The listing builds one solid part. Answer for the finished solid, in the listing's coordinates (mm). A direction names the side the tool comes from. Coordinates: 2 decimals unless noted, no trailing zeros. Write each loop counter-clockwise with the first axis right and the second up, starting at its lowest first coordinate (ties: lowest second). Pieces come first, ordered by that corner, then holes.
from build123d import *

# Parameters (mm, degrees)
SKETCH1_W               = 70.4
SKETCH1_H               = 2
BOSS_EXTRUDE2_DEPTH     = 10
SKETCH2_W               = 2
SKETCH2_H               = 55
BOSS_EXTRUDE3_DEPTH     = 10
SKETCH3_W               = 19
SKETCH3_H               = 3
BOSS_EXTRUDE4_DEPTH     = 2
SKETCH4_W               = 15
SKETCH4_H               = 10
CUT_EXTRUDE2_DEPTH      = 2
SKETCH5_W               = 2
SKETCH5_H               = 3
BOSS_EXTRUDE5_DEPTH     = 1
SKETCH6_W               = 2
SKETCH6_H               = 3
BOSS_EXTRUDE6_DEPTH     = 1
SKETCH7_W               = 57
SKETCH7_H               = 2
BOSS_EXTRUDE7_DEPTH     = 6.6
SKETCH8_W               = 57
SKETCH8_H               = 2
BOSS_EXTRUDE8_DEPTH     = 6.6
BOSS_EXTRUDE9_DEPTH     = 5
SKETCH12_W              = 2
SKETCH12_H              = 5
SKETCH12_H_2            = 40
SKETCH12_H_3            = 30
BOSS_EXTRUDE10_DEPTH    = 20
BOSS_EXTRUDE11_DEPTH    = 3
SKETCH14_W              = 0.5
SKETCH14_H              = 9
CUT_EXTRUDE3_DEPTH      = 3
SKETCH15_W              = 38.4
SKETCH15_H              = 45
CUT_EXTRUDE4_DEPTH      = 3
BOSS_EXTRUDE12_DEPTH    = 0.5
SKETCH17_R              = 1.8
SKETCH17_W              = 3
SKETCH17_H              = 5
CUT_EXTRUDE6_DEPTH      = 3
CUT_EXTRUDE8_DEPTH      = 32
CUT_EXTRUDE8_DEPTH_BACK = 49
SKETCH19_W              = 94.558020587
SKETCH19_H              = 51.225034616
CUT_EXTRUDE9_DEPTH      = 93
CUT_EXTRUDE9_DEPTH_BACK = 18
SKETCH20_W              = 91.945359737
SKETCH20_H              = 40.424662202
SKETCH21_W              = 45
SKETCH21_H              = 3
BOSS_EXTRUDE14_DEPTH    = 2.5
SKETCH22_W              = 2.5
SKETCH22_H              = 45
BOSS_EXTRUDE15_DEPTH    = 8
SKETCH23_R              = 1.8
CUT_EXTRUDE10_DEPTH     = 10


with BuildPart() as part:
    # Sketch1 → Boss-Extrude2 (new body)
    with BuildSketch(Plane(origin=(0, 0, 0), x_dir=(1, 0, 0), z_dir=(0, 1, 0))):
        with Locations((35.2, 1)):
            Rectangle(SKETCH1_W, SKETCH1_H)
    extrude(amount=BOSS_EXTRUDE2_DEPTH)

    # Sketch2 → Boss-Extrude3 (add)
    with BuildSketch(Plane(origin=(0, 10, 0), x_dir=(1, 0, 0), z_dir=(0, 1, 0))):
        with Locations((1, 29.5)):
            Rectangle(SKETCH2_W, SKETCH2_H)
        with Locations((69.4, 29.5)):
            Rectangle(SKETCH2_W, SKETCH2_H)
    extrude(amount=-BOSS_EXTRUDE3_DEPTH)

    # Sketch3 → Boss-Extrude4 (add)
    with BuildSketch(Plane.XY):
        with Locations((35.2, 11.5)):
            Rectangle(SKETCH3_W, SKETCH3_H)
    extrude(amount=-BOSS_EXTRUDE4_DEPTH)

    # Sketch4 → Cut-Extrude2 (cut)
    with BuildSketch(Plane.XY):
        with Locations((35.2, 5)):
            Rectangle(SKETCH4_W, SKETCH4_H)
    extrude(amount=-CUT_EXTRUDE2_DEPTH, mode=Mode.SUBTRACT)

    # Sketch5 → Boss-Extrude5 (add)
    with BuildSketch(Plane.ZY.offset(-25.7)):
        with Locations((-1, 11.5)):
            Rectangle(SKETCH5_W, SKETCH5_H)
    extrude(amount=BOSS_EXTRUDE5_DEPTH)

    # Sketch6 → Boss-Extrude6 (add)
    with BuildSketch(Plane(origin=(44.7, 0, 0), x_dir=(0, 0, -1), z_dir=(1, 0, 0))):
        with Locations((1, 11.5)):
            Rectangle(SKETCH6_W, SKETCH6_H)
    extrude(amount=BOSS_EXTRUDE6_DEPTH)

    # Sketch7 → Boss-Extrude7 (add)
    with BuildSketch(Plane.ZY):
        with Locations((-28.5, 1)):
            Rectangle(SKETCH7_W, SKETCH7_H)
    extrude(amount=BOSS_EXTRUDE7_DEPTH)

    # Sketch8 → Boss-Extrude8 (add)
    with BuildSketch(Plane(origin=(70.4, 0, 0), x_dir=(0, 0, -1), z_dir=(1, 0, 0))):
        with Locations((28.5, 1)):
            Rectangle(SKETCH8_W, SKETCH8_H)
    extrude(amount=BOSS_EXTRUDE8_DEPTH)

    # Sketch10 → Boss-Extrude9 (add)
    with BuildSketch(Plane(origin=(0, 0, -57), x_dir=(-1, 0, 0), z_dir=(0, 0, -1))):
        Polygon((-2, 10), (-2, 0), (6.6, 0), (6.6, 2), (0, 2), (0, 10), align=None)
        Polygon((-77, 0), (-68.4, 0), (-68.4, 10), (-70.4, 10), (-70.4, 2), (-77, 2), align=None)
    extrude(amount=BOSS_EXTRUDE9_DEPTH)

    # Sketch12 → Boss-Extrude10 (add)
    with BuildSketch(Plane(origin=(0, 10, 0), x_dir=(1, 0, 0), z_dir=(0, 1, 0))):
        with Locations((1, 59.5)):
            Rectangle(SKETCH12_W, SKETCH12_H)
        with Locations((1, 37)):
            Rectangle(SKETCH12_W, SKETCH12_H_2)
        with Locations((69.4, 42)):
            Rectangle(SKETCH12_W, SKETCH12_H_3)
        with Locations((69.4, 59.5)):
            Rectangle(SKETCH12_W, SKETCH12_H)
    extrude(amount=BOSS_EXTRUDE10_DEPTH)

    # Sketch13 → Boss-Extrude11 (add)
    with BuildSketch(Plane(origin=(0, 30, 0), x_dir=(1, 0, 0), z_dir=(0, 1, 0))):
        Polygon((0, 17), (35.2, 17), (35.2, 27), (70.4, 27), (70.4, 62), (0, 62), align=None)
    extrude(amount=BOSS_EXTRUDE11_DEPTH)

    # Sketch14 → Cut-Extrude3 (cut)
    with BuildSketch(Plane(origin=(0, 33, 0), x_dir=(1, 0, 0), z_dir=(0, 1, 0))):
        with Locations((11.7, 51)):
            Rectangle(SKETCH14_W, SKETCH14_H)
        with Locations((11.7, 38)):
            Rectangle(SKETCH14_W, SKETCH14_H)
        with Locations((11.7, 25.5)):
            Rectangle(SKETCH14_W, SKETCH14_H)
        with Locations((58.2, 51)):
            Rectangle(SKETCH14_W, SKETCH14_H)
        with Locations((58.2, 38)):
            Rectangle(SKETCH14_W, SKETCH14_H)
    extrude(amount=-CUT_EXTRUDE3_DEPTH, mode=Mode.SUBTRACT)

    # Sketch15 → Cut-Extrude4 (cut)
    with BuildSketch(Plane(origin=(0, 33, 0), x_dir=(1, 0, 0), z_dir=(0, 1, 0))):
        with Locations((35.2, 39.5)):
            Rectangle(SKETCH15_W, SKETCH15_H)
    extrude(amount=-CUT_EXTRUDE4_DEPTH, mode=Mode.SUBTRACT)

    # Sketch16 → Boss-Extrude12 (add)
    with BuildSketch(Plane.XY):
        Polygon((-6.6, 0), (27.7, 0), (27.7, 10), (42.7, 10), (42.7, 0), (77, 0), (77, 2), (70.4, 2), (70.4, 10), (45.7, 10), (45.7, 13), (24.7, 13), (24.7, 10), (0, 10), (0, 2), (-6.6, 2), align=None)
    extrude(amount=BOSS_EXTRUDE12_DEPTH)

    # Sketch17 → Cut-Extrude6 (cut)
    with BuildSketch(Plane(origin=(0, 2, 0), x_dir=(1, 0, 0), z_dir=(0, 1, 0))):
        with Locations(Location((-3.3, 55, 0), (0, 0, 270))):
            Circle(SKETCH17_R)
        with Locations(Location((73.7, 55, 0), (0, 0, 270))):
            Circle(SKETCH17_R)
        with Locations(Location((-3.3, 6.5, 0), (0, 0, 270))):
            Circle(SKETCH17_R)
        with Locations(Location((73.7, 6.5, 0), (0, 0, 270))):
            Circle(SKETCH17_R)
        with Locations(Location((-3.3, 30.75, 0), (0, 0, 270))):
            Circle(SKETCH17_R)
        with Locations(Location((73.7, 30.75, 0), (0, 0, 270))):
            Circle(SKETCH17_R)
        with Locations((-3.3, 14.5)):
            Rectangle(SKETCH17_W, SKETCH17_H)
        with Locations((73.7, 14.5)):
            Rectangle(SKETCH17_W, SKETCH17_H)
    extrude(amount=-CUT_EXTRUDE6_DEPTH, mode=Mode.SUBTRACT)

    # Sketch19 → Cut-Extrude8 (cut, two sides: drawn at the far end of the back side and taken through both)
    with BuildSketch(Plane(origin=(70.4, 0, 0), x_dir=(0, 0, -1), z_dir=(1, 0, 0)).offset(-CUT_EXTRUDE8_DEPTH_BACK)):
        with Locations((14.720989707, 7.387482692)):
            Rectangle(SKETCH19_W, SKETCH19_H)
    extrude(amount=CUT_EXTRUDE8_DEPTH + CUT_EXTRUDE8_DEPTH_BACK, mode=Mode.SUBTRACT)

    # Sketch20 → Cut-Extrude9 (cut, two sides: drawn at the far end of the back side and taken through both)
    with BuildSketch(Plane(origin=(2, 0, 0), x_dir=(0, 0, -1), z_dir=(1, 0, 0)).offset(-CUT_EXTRUDE9_DEPTH_BACK)):
        with Locations((16.027320132, 9.787668899)):
            Rectangle(SKETCH20_W, SKETCH20_H)
    extrude(amount=CUT_EXTRUDE9_DEPTH + CUT_EXTRUDE9_DEPTH_BACK, mode=Mode.SUBTRACT)

    # Sketch21 → Boss-Extrude14 (add)
    with BuildSketch(Plane.ZY):
        with Locations((-39.5, 31.5)):
            Rectangle(SKETCH21_W, SKETCH21_H)
    extrude(amount=BOSS_EXTRUDE14_DEPTH)

    # Sketch22 → Boss-Extrude15 (add)
    with BuildSketch(Plane.XZ.offset(-30)):
        with Locations((-1.25, -39.5)):
            Rectangle(SKETCH22_W, SKETCH22_H)
    extrude(amount=BOSS_EXTRUDE15_DEPTH)

    # Sketch23 → Cut-Extrude10 (cut)
    with BuildSketch(Plane(origin=(0, 0, 0), x_dir=(0, 0, -1), z_dir=(1, 0, 0))):
        with Locations((27, 26)):
            Circle(SKETCH23_R)
        with Locations((52, 26)):
            Circle(SKETCH23_R)
    extrude(amount=-CUT_EXTRUDE10_DEPTH, mode=Mode.SUBTRACT)


solid = part.part
Q1. Given pin 1 (6 mm diameter, centred on y = 23, z = -40, fed in from +X); pin 2 (2 mm diameter, centred on y = 26, z = -52, fed in from +X); pin 3 (4 mm diameter, centred on x = 3, z = -31, fed in from -Y), each flat-ended and moving along its own axis, determine where each tip first touches the part or whether it passes through.
Answers below:
pin 1: stops at x = 0
pin 2: passes through
pin 3: stops at y = 30
Q2. The part is cut by section B-B, the plane z = -39. Write down the section's boundary in (x, y), then the cut area to 3 significant figures.
Answers below:
outline: (-2.5, 22) - (0, 22) - (0, 30) - (11.45, 30) - (11.45, 33) - (-2.5, 33) - close; (11.95, 30) - (16, 30) - (16, 33) - (11.95, 33) - close
area: 74.0 mm2
Q3. The part is cut by section A-A, the plane z = -52. Write down the section's boundary in (x, y), then the cut area to 3 significant figures.
Answers below:
outline: (-2.5, 22) - (0, 22) - (0, 24.2) - (-2.5, 24.2) - close; (-2.5, 27.8) - (0, 27.8) - (0, 30) - (11.45, 30) - (11.45, 33) - (-2.5, 33) - close; (11.95, 30) - (16, 30) - (16, 33) - (11.95, 33) - close
area: 65.0 mm2
Q4. Determine the mould class of faces 1 (the face through (16, 32, -39)), 2 (the face through (7, 33, -40)), 3 (the face through (11.45, 32, -38)) for opening direction X: released by +X, released by -X, zero draft, split by the parting line, or undercut.
Answers below:
face 1: released by +X
face 2: zero draft
face 3: undercut
Q5. Which of the six approach directions +Z, -Z, +X, -X, +Y, -Y give full straight-line access (tool end or side, diameter ignored) to faces 4 (the face through (8, 30, -40)), 5 (the face through (-1.232, 27.785, -51.766)), 6 (the face through (11.95, 32, -51))?
Answers below:
face 4: +Z, -Z, +X, -Y
face 5: +X, -X
face 6: +Y, -Y
Q6. The part is cut by section C-C, the plane z = -20. Write down the section's boundary in (x, y), then the cut area to 3 significant figures.
Answers below:
outline: (-2.5, 22) - (0, 22) - (0, 30) - (16, 30) - (16, 33) - (-2.5, 33) - close
area: 75.5 mm2
Q7. The part is cut by section D-D, the plane y = 23.5. Write down the section's boundary in (x, z), then the cut area to 4 significant figures.
Answers below:
outline: (-2.5, -62) - (0, -62) - (0, -17) - (-2.5, -17) - close
area: 112.5 mm2
Q8. Find the intervals of material crossed by probe 1 along Z at (x, y) = (11.5, 30.75); probe 2 along Y at (x, z) = (-0.9, -27); probe 3 along X at (y, z) = (32.5, -39.5), in increasing order.
Answers below:
probe 1: z = -62 to -55.5, -46.5 to -42.5, -33.5 to -30, -21 to -17
probe 2: y = 22 to 24.2, 27.8 to 33
probe 3: x = -2.5 to 11.45, 11.95 to 16
